Input: part model. Units: mm. Frame: model coordinates. A direction names the side the tool comes from. Round coordinates to 2 decimals unless told otherwise and drop trailing zeros. Loops run counter-clockwise (first coordinate to the right, second up) from the corner with the lowest first, then second, coordinate; pieces in that order, holes last. Notation, with made-up numbers: (-29, -39) -> (-6, -39) arc R31 cw to (-6, -9) -> close; hole circle Ø10 at (81, -6). An arc over 180 degrees is marked (long way). Answer as a JSON object with one key per item and string values.
```python
from build123d import *

# Parameters (mm, degrees)
SKETCH1_W           = 12.7
SKETCH1_H           = 25.4
SKETCH1_R           = 1.905
BOSS_EXTRUDE1_DEPTH = 6.35


with BuildPart() as part:
    # Sketch1 → Boss-Extrude1 (new body)
    with BuildSketch(Plane(origin=(0, 0, 0), x_dir=(0, 0, -1), z_dir=(1, 0, 0))):
        Polygon((0, 14.9225), (0, 6.35), (0, 0), (6.35, 0), (18.7325, 0), (18.7325, 6.35), (35.8775, 6.35), (35.8775, 0), (53.0225, 0), (53.0225, 6.35), (70.1675, 6.35), (70.1675, 0), (82.55, 0), (88.9, 0), (88.9, 6.35), (88.9, 14.9225), (82.55, 14.9225), (82.55, 32.0675), (88.9, 32.0675), (88.9, 49.2125), (82.55, 49.2125), (82.55, 66.3575), (88.9, 66.3575), (88.9, 83.5025), (82.55, 83.5025), (82.55, 100.6475), (88.9, 100.6475), (88.9, 117.7925), (82.55, 117.7925), (82.55, 134.9375), (88.9, 134.9375), (88.9, 152.0825), (82.55, 152.0825), (82.55, 169.2275), (88.9, 169.2275), (88.9, 186.3725), (82.55, 186.3725), (82.55, 203.5175), (88.9, 203.5175), (88.9, 220.6625), (82.55, 220.6625), (82.55, 237.8075), (88.9, 237.8075), (88.9, 254.9525), (82.55, 254.9525), (82.55, 272.0975), (88.9, 272.0975), (88.9, 289.2425), (82.55, 289.2425), (82.55, 306.3875), (88.9, 306.3875), (88.9, 323.5325), (82.55, 323.5325), (82.55, 340.6775), (88.9, 340.6775), (88.9, 349.25), (70.1675, 349.25), (70.1675, 355.6), (53.0225, 355.6), (53.0225, 349.25), (35.8775, 349.25), (35.8775, 355.6), (18.7325, 355.6), (18.7325, 349.25), (6.35, 349.25), (0, 349.25), (0, 340.6775), (6.35, 340.6775), (6.35, 334.518000001), (6.35, 329.692000001), (6.35, 323.5325), (0, 323.5325), (0, 306.3875), (6.35, 306.3875), (6.35, 289.2425), (0, 289.2425), (0, 272.0975), (6.35, 272.0975), (6.35, 254.9525), (0, 254.9525), (0, 237.8075), (6.35, 237.8075), (6.35, 220.6625), (0, 220.6625), (0, 203.5175), (6.35, 203.5175), (6.35, 186.3725), (0, 186.3725), (0, 169.2275), (6.35, 169.2275), (6.35, 152.0825), (0, 152.0825), (0, 134.9375), (6.35, 134.9375), (6.35, 117.7925), (0, 117.7925), (0, 100.6475), (6.35, 100.6475), (6.35, 83.5025), (0, 83.5025), (0, 66.3575), (6.35, 66.3575), (6.35, 49.2125), (0, 49.2125), (0, 32.0675), (6.35, 32.0675), (6.35, 25.907999999), (6.35, 21.081999999), (6.35, 14.9225), align=None)
        with Locations((69.85, 177.8)):
            Rectangle(SKETCH1_W, SKETCH1_H, mode=Mode.SUBTRACT)
        with Locations((69.85, 203.2)):
            Circle(SKETCH1_R, mode=Mode.SUBTRACT)
    extrude(amount=BOSS_EXTRUDE1_DEPTH)


solid = part.part
```
1) Draft query along Y for faces 1 (the face through (3, 355.6, -62)), 2 (the face through (3, 161, -6.35)), 3 (the face through (3, 178, 0)). Return one class per face: +Y half, -Y half, draft (parallel to the pull), parting line (faces both ways), or undercut.
Output:
{"face 1": "+Y half", "face 2": "undercut", "face 3": "draft"}
2) Contact query for flat-ended pins moving along their axis: P1, Ø2, axis at x = 2.5, y = 88.5, coming from the -Z side; P2, Ø1.5, axis at x = 4.5, z = -41, coming from the +Y side; P3, Ø3, axis at x = 4, y = 124, coming from the +Z side; P4, Ø3, axis at y = 203.2, z = -69.85, coming from the +X side. Output: stop coordinate, or through.
Output:
{"P1": "stops at z = -82.55", "P2": "stops at y = 349.25", "P3": "stops at z = -6.35", "P4": "passes through"}
3) Section A-A, the plane z = -29. Output: boundary loops of the cut face in (x, y), plus the area to 3 significant figures.
Output:
{"outline": "(0, 6.35) -> (6.35, 6.35) -> (6.35, 355.6) -> (0, 355.6) -> close", "area": "2,220 mm^2"}
4) Section B-B, the plane x = 1.75. Count the separate pieces of the cut face and the enclosed holes in it, plus the area to 3 significant figures.
Output:
{"separate pieces": "1", "enclosed holes": "2", "area": "28,500 mm^2"}
5) Ray query, probe 1 along Y at (x, z) = (4.5, -69.85) (3 decimals); probe 2 along Z at (x, y) = (1.5, 203.2) (3 decimals); probe 3 along Y at (x, z) = (4.75, -74). Return the intervals inside material, ascending.
Output:
{"probe 1": "y = 6.35 to 165.1, 190.5 to 201.295, 205.105 to 355.6", "probe 2": "z = -82.55 to -71.755, -67.945 to -6.35", "probe 3": "y = 0 to 165.1, 190.5 to 349.25"}
6) Reachability of faces 4 (the face through (3, 165.1, -70)), 5 (the face through (3, 352, -35.878)), 6 (the face through (3, 263, -82.55)) from +Z, -Z, +X, -X, +Y, -Y: full face, straight path, thin tool, end or side. Return the list, or none.
Output:
{"face 4": "+X, -X", "face 5": "+X, -X, +Y", "face 6": "-Z, +X, -X"}
